Read the model definition and answer for the solid it produces. Units are mm, in the model's axes. A direction names the side the tool comes from. Round coordinates to 2 decimals unless told otherwise and drop trailing zeros. Order: outer loops, then holes, each group sorted by start corner. A loop starts at its lowest first (then second) coordinate and runs counter-clockwise, first axis right, second up. Notation, with made-up numbers: (77.25, -38.5) - (89.25, -38.5) arc R11 cw to (89.25, -32.5) - close; hole circle Ø8 at (45.5, 0). An arc over 180 degrees is marked (long way). Answer as a JSON object with one key per item and string values. Group by question number.
Q1. The mould has two halves that part along Y. Classify faces 1 (the flat face through (-59, 4, 24.5)), 2 (the flat face through (-67.49, 3, 25)), 3 (the flat face through (-38, -1, 0)): pulls with the +Y half, pulls with the -Y half, needs draft (parallel to the pull), parting line crosses it, or undercut.
Q2. A tool of negligible diameter and unlimited length cuts with its end or side. For faces 4 (the flat face through (-51.49, 3, 25)), 5 (the flat face through (-59, 6, -24.5)), 6 (the flat face through (-59, 4.9, 24)), from which of +Z, -Z, +X, -X, +Y, -Y can it reach the whole face along a straight path? Write none if from no direction.
Q3. A cutting plane is placed at B-B on y = 5.75. Determine the outline of the cut face in (x, z).
Q4. A cutting plane is placed at D-D on x = -15. Determine the outline of the cut face in (y, z).
Q5. Given pin 1 Ø4 at (y, z) = (2.5, 24.5) entering from +X; pin 2 Ø3 at (x, z) = (3, -28) entering from +Y; pin 3 Ø2.5 at (y, z) = (3, 25) entering from -X; pin 4 Ø3 at (x, z) = (-24, 23) entering from +Y, each flat-ended and moving along its own axis, determine where each tip first touches the part or whether it passes through.
Q6. A cutting plane is placed at A-A on z = -28. Determine the outline of the cut face in (x, y).
Q7. Consider line 1 (Z direction, x = 3, y = -0.25); line 2 (Z direction, x = -15, y = -0.2); line 3 (X direction, y = -0.5, z = 6). Determine where each line is inside the solid, lowest interval first.
Q8. A cutting plane is placed at C-C on x = 3. Determine the outline of the cut face in (y, z), and give its area (3 significant figures).
```python
from build123d import *

# Parameters (mm, degrees)
SKETCH009_W  = 84.9897948557
SKETCH009_H  = 61
SKETCH009_R  = 1.55
PAD005_DEPTH = 1
CHAMFER_SIZE = 0.5
PAD007_DEPTH = 16


with BuildPart() as part:
    # Sketch009 → Pad005 (new body)
    with BuildSketch(Plane.XZ):
        with Locations((-36.9948974278, 0)):
            Rectangle(SKETCH009_W, SKETCH009_H)
        with Locations((3, -28)):
            Circle(SKETCH009_R, mode=Mode.SUBTRACT)
        with Locations((3, 28)):
            Circle(SKETCH009_R, mode=Mode.SUBTRACT)
        with Locations((-76.9897948557, 28)):
            Circle(SKETCH009_R, mode=Mode.SUBTRACT)
        with Locations((-76.9897948557, -28)):
            Circle(SKETCH009_R, mode=Mode.SUBTRACT)
        with Locations((-15, 5)):
            Circle(SKETCH009_R, mode=Mode.SUBTRACT)
        with Locations((-34, 5)):
            Circle(SKETCH009_R, mode=Mode.SUBTRACT)
    extrude(amount=PAD005_DEPTH)

    # Chamfer
    chamfer_edges = [part.edges().sort_by_distance(p)[0] for p in [
        (-78.539795, -1, -28),
        (-16.55, -1, 5),
        (1.45, -1, 28),
        (1.45, -1, -28),
        (-78.539795, -1, 28),
        (-35.55, -1, 5),
    ]]
    chamfer(chamfer_edges, length=CHAMFER_SIZE)

    # Sketch011 (on DatumPlane) → Pad007 (join)
    with BuildSketch(Plane(origin=(-51.4897948557, 0, 0), x_dir=(0, 0, -1), z_dir=(-1, 0, 0))):
        Polygon((-27.5, 1), (29.5, 1), (29.5, -6.9), (24.5, -6.9), (24.5, -4.9), (26.5, -4.9), (26.5, -3), (24.5, -3), (24.5, 0), (-22.5, 0), (-22.5, -3), (-24.5, -3), (-24.5, -4.9), (-22.5, -4.9), (-22.5, -6.9), (-27.5, -6.9), align=None)
    extrude(amount=PAD007_DEPTH)


solid = part.part
```
Result set:
{
 "1": {"face 1": "undercut", "face 2": "needs draft", "face 3": "pulls with the -Y half"},
 "2": {"face 4": "+Z, -Z, +X, +Y", "face 5": "+X, -X, +Y", "face 6": "+X, -X"},
 "3": {"outline": "(-67.49, -29.5) - (-51.49, -29.5) - (-51.49, -24.5) - (-67.49, -24.5) - close; (-67.49, 22.5) - (-51.49, 22.5) - (-51.49, 27.5) - (-67.49, 27.5) - close"},
 "4": {"outline": "(-1, -30.5) - (0, -30.5) - (0, 3.45) - (-0.5, 3.45) - (-1, 2.95) - close; (-1, 7.05) - (-0.5, 6.55) - (0, 6.55) - (0, 30.5) - (-1, 30.5) - close"},
 "5": {"pin 1": "stops at x = -51.49", "pin 2": "passes through", "pin 3": "stops at x = -67.49", "pin 4": "stops at y = 0"},
 "6": {"outline": "(-79.49, -1) - (-79.04, -1) - (-78.54, -0.5) - (-78.54, 0) - (-79.49, 0) - close; (-75.44, -0.5) - (-74.94, -1) - (0.95, -1) - (1.45, -0.5) - (1.45, 0) - (-51.49, 0) - (-51.49, 6.9) - (-67.49, 6.9) - (-67.49, 0) - (-75.44, 0) - close; (4.55, -0.5) - (5.05, -1) - (5.5, -1) - (5.5, 0) - (4.55, 0) - close"},
 "7": {"line 1": "z = -30.5 to -29.55, -26.45 to 26.45, 29.55 to 30.5", "line 2": "z = -30.5 to 3.45, 6.55 to 30.5", "line 3": "x = -79.49 to -35.18, -32.82 to -16.18, -13.82 to 5.5"},
 "8": {"outline": "(-1, -30.5) - (0, -30.5) - (0, -29.55) - (-0.5, -29.55) - (-1, -30.05) - close; (-1, -25.95) - (-0.5, -26.45) - (0, -26.45) - (0, 26.45) - (-0.5, 26.45) - (-1, 25.95) - close; (-1, 30.05) - (-0.5, 29.55) - (0, 29.55) - (0, 30.5) - (-1, 30.5) - close", "area": "54.3 mm²"}
}
